Input: part model. Units: mm. Frame: model coordinates. A direction names the side the tool comes from. Coordinates: 2 decimals unless noted, no trailing zeros. Loops run counter-clockwise (first coordinate to the right, second up) from the corner with the lowest first, then second, coordinate; pieces in that order, holes last. Notation, with made-up numbers: M -38,-28.75 L -13,-28.75 A10 ccw -13,-15.75 Z; hole C 30,19.25 d11. An arc over 180 degrees is marked long. Use a Markdown table: item, result. Add a question column.
1. Section D-D on z = 5. State how many separate pieces and enclosed holes the cut face has, then the cut area to 3 significant figures.
2. Line query: L1, parallel to X at y = -28, z = 2; L2, parallel to X at y = 21, z = 0.75; L3, parallel to X at y = -3.5, z = 1.5. Output: solid intervals per line, ascending. Write a range as [from, to].
3. Pin query (flat end, axial travel): pin 1 (4.5 mm diameter, centred on x = -11.5, y = 11.5, fed in from +Z); pin 2 (1 mm diameter, centred on y = -40.5, z = 4.5, fed in from -X); pin 3 (3 mm diameter, centred on x = -16, z = 5, fed in from -Y). Return the tip coordinate at first contact, or that it passes through.
4. Section C-C on y = -3. Output: boundary loops of the cut face in (x, z).
5. Section B-B on y = -27. Output: boundary loops of the cut face in (x, z), then the cut area to 3 significant figures.
6. Set-up query: faces 1 (the flat face through (18.213, 25.756, 3.219)), 2 (the cylindrical face through (-8.88, -10.67, 5.12)). Return all of +Z, -Z, +X, -X, +Y, -Y with unobstructed straight access to the full face (end or side cutting, diameter ignored); none if empty.
7. Section A-A on x = 0. Output: boundary loops of the cut face in (y, z).
```python
from build123d import *

# Parameters (mm, degrees)
SKETCH1_R                        = 50.8
BOSS_EXTRUDE1_DEPTH              = 6.35
SKETCH2_R                        = 11.43
CUT_EXTRUDE1_DEPTH               = 7.35
CBORE_FOR_M2_5_SHCS1_D           = 2.7
CBORE_FOR_M2_5_SHCS1_DEPTH       = 10.16
CBORE_FOR_M2_5_SHCS1_CBORE_D     = 5.5
CBORE_FOR_M2_5_SHCS1_CBORE_DEPTH = 2.5
CBORE_FOR_M2_5_SHCS1_TIP         = 0.811161836
F_6_CLEARANCE_HOLE1_D            = 3.6576
F_6_CLEARANCE_HOLE1_DEPTH        = 10.16
F_6_CLEARANCE_HOLE1_TIP          = 1.0988539
CUT_EXTRUDE2_DEPTH               = 7.35
FILLET2_R                        = 3.175
CIRPATTERN1_COUNT                = 3
FILLET2_OF_CIRPATTERN1_R         = 3.175


with BuildPart() as part:
    # Sketch1 → Boss-Extrude1 (new body)
    with BuildSketch(Plane.XY):
        Circle(SKETCH1_R)
    extrude(amount=BOSS_EXTRUDE1_DEPTH)

    # Sketch2 → Cut-Extrude1 (cut, through all)
    with BuildSketch(Plane.XY.offset(6.35)):
        Circle(SKETCH2_R)
    extrude(amount=-CUT_EXTRUDE1_DEPTH, mode=Mode.SUBTRACT)

    # CBORE for M2.5 SHCS1
    with Locations(Plane.XY.offset(6.35)):
        with Locations((0, 0), (11.5, 11.5), (-11.5, -11.5), (-11.5, 11.5), (11.5, -11.5)):
            CounterBoreHole(CBORE_FOR_M2_5_SHCS1_D / 2, CBORE_FOR_M2_5_SHCS1_CBORE_D / 2, CBORE_FOR_M2_5_SHCS1_CBORE_DEPTH, depth=CBORE_FOR_M2_5_SHCS1_DEPTH)
            with Locations((0, 0, -(CBORE_FOR_M2_5_SHCS1_DEPTH + CBORE_FOR_M2_5_SHCS1_TIP / 2))):  # 118° drill point
                Cone(0, CBORE_FOR_M2_5_SHCS1_D / 2, CBORE_FOR_M2_5_SHCS1_TIP, mode=Mode.SUBTRACT)

    # #6 Clearance Hole1
    with Locations(Plane.XY.offset(6.35)):
        with Locations((-38.1, 21.997045256), (0, -43.994090512), (38.1, 21.997045256)):
            Hole(F_6_CLEARANCE_HOLE1_D / 2, depth=F_6_CLEARANCE_HOLE1_DEPTH)
            with Locations((0, 0, -(F_6_CLEARANCE_HOLE1_DEPTH + F_6_CLEARANCE_HOLE1_TIP / 2))):  # 118° drill point
                Cone(0, F_6_CLEARANCE_HOLE1_D / 2, F_6_CLEARANCE_HOLE1_TIP, mode=Mode.SUBTRACT)

    # Sketch10 → Cut-Extrude2 (cut, through all)
    with BuildSketch(Plane.XY.offset(6.35)):
        with BuildLine():
            Line((14.664933069, 20.738846113), (21.997399604, 31.108269169))
            ThreePointArc((21.997399604, 31.108269169), (0, 38.1), (-21.997399604, 31.108269169))
            Line((-21.997399604, 31.108269169), (-14.664933069, 20.738846113))
            ThreePointArc((-14.664933069, 20.738846113), (0, 25.4), (14.664933069, 20.738846113))
        make_face()
    cut_extrude2 = extrude(amount=-CUT_EXTRUDE2_DEPTH, mode=Mode.SUBTRACT)

    # Fillet2
    fillet2_edges = [part.edges().sort_by_distance(p)[0] for p in [
        (-21.997399604, 31.108269169, 3.175),
        (21.997399604, 31.108269169, 3.175),
        (14.664933069, 20.738846113, 3.175),
        (-14.664933069, 20.738846113, 3.175),
    ]]
    fillet(fillet2_edges, radius=FILLET2_R)

    # CirPattern1: Cut-Extrude2 ×3 about axis
    cirpattern1_axis = Axis((0, 0, 0), (0, 0, 1))
    for i in range(1, CIRPATTERN1_COUNT):
        add(cut_extrude2.rotate(cirpattern1_axis, i * 360 / CIRPATTERN1_COUNT), mode=Mode.SUBTRACT)

    # Fillet2 of CirPattern1
    fillet2_of_cirpattern1_edges = [part.edges().sort_by_distance(p)[0] for p in [
        (-15.941851566, -34.604441458, 3.175),
        (-37.93925117, 3.49617229, 3.175),
        (-25.292834113, 2.330781526, 3.175),
        (-10.627901044, -23.069627639, 3.175),
        (37.93925117, 3.49617229, 3.175),
        (15.941851566, -34.604441458, 3.175),
        (10.627901044, -23.069627639, 3.175),
        (25.292834113, 2.330781526, 3.175),
    ]]
    fillet(fillet2_of_cirpattern1_edges, radius=FILLET2_OF_CIRPATTERN1_R)


solid = part.part
```
Answers below:
| question | item | result |
|---|---|---|
| 1 | separate pieces | 1 |
| 1 | enclosed holes | 11 |
| 1 | area | 6,110 mm² |
| 2 | L1 | x = [-42.39, -25.84], [-12.9, 12.9], [25.84, 42.39] |
| 2 | L2 | x = [-46.26, -39.63], [-36.57, 36.57], [39.63, 46.26] |
| 2 | L3 | x = [-50.68, -37.94], [-25.16, -10.88], [10.88, 25.16], [37.94, 50.68] |
| 3 | pin 1 | stops at z = 3.85 |
| 3 | pin 2 | stops at x = -31.32 |
| 3 | pin 3 | stops at y = -48.69 |
| 4 | outline | M -50.71,0 L -37.98,0 L -37.98,6.35 L -50.71,6.35 Z; M -25.22,0 L -11.03,0 L -11.03,6.35 L -25.22,6.35 Z; M 11.03,0 L 25.22,0 L 25.22,6.35 L 11.03,6.35 Z; M 37.98,0 L 50.71,0 L 50.71,6.35 L 37.98,6.35 Z |
| 5 | outline | M -43.03,0 L -26.88,0 L -26.88,6.35 L -43.03,6.35 Z; M -12.44,0 L 12.44,0 L 12.44,6.35 L -12.44,6.35 Z; M 26.88,0 L 43.03,0 L 43.03,6.35 L 26.88,6.35 Z |
| 5 | area | 363 mm² |
| 6 | face 1 | +Z, -Z |
| 6 | face 2 | +Z |
| 7 | outline | M -50.8,0 L -45.82,0 L -45.82,6.35 L -50.8,6.35 Z; M -42.17,0 L -11.43,0 L -11.43,6.35 L -42.17,6.35 Z; M 11.43,0 L 25.4,0 L 25.4,6.35 L 11.43,6.35 Z; M 38.1,0 L 50.8,0 L 50.8,6.35 L 38.1,6.35 Z |
